from build123d import *

# Parameters (mm, degrees)
SKETCH2_R           = 90
SKETCH1_R           = 90
SHELL1_T            = -2
CUT_EXTRUDE1_START  = -50
SKETCH4_R           = 90
CUT_EXTRUDE1_DEPTH  = 50
FILLET1_R           = 10
SKETCH5_R           = 88
BOSS_EXTRUDE1_DEPTH = 2


with BuildPart() as part:
    # Sketch2 → Loft1 section 0
    with BuildSketch(Plane(origin=(0, 100, 0), x_dir=(1, 0, 0), z_dir=(0, 1, 0))):
        Circle(SKETCH2_R)
    # Sketch1 → Loft1 section 1
    with BuildSketch(Plane(origin=(0, 0, 0), x_dir=(1, 0, 0), z_dir=(0, 1, 0))):
        Circle(SKETCH1_R)
    loft()

    # Shell1
    shell1_openings = [part.faces().sort_by_distance(p)[0] for p in [
        (0, 100, 0),
    ]]
    offset(amount=SHELL1_T, openings=shell1_openings, kind=Kind.INTERSECTION)

    # Sketch4 → Cut-Extrude1 (cut)
    with BuildSketch(Plane(origin=(0, 100, 0), x_dir=(1, 0, 0), z_dir=(0, 1, 0)).offset(CUT_EXTRUDE1_START)):
        with Locations(Location((0, 0, 0), (0, 0, 270))):
            Circle(SKETCH4_R)
    extrude(amount=CUT_EXTRUDE1_DEPTH, mode=Mode.SUBTRACT)

    # Fillet1
    # the kernel refuses this fillet: 10 mm, written as the material it takes off along each edge
    with BuildSketch(Plane(origin=(0, 50, 0), x_dir=(1, 0, 0), z_dir=(0, 0, -1))) as fillet1_piece_1:
        with BuildLine():
            CenterArc((80, 6), FILLET1_R, 323.130102354, 36.869897646)
            Line((88, 0), (88.16, -0.12))
            ThreePointArc((88.16, -0.12), (89, -0.2), (90, -0.2))
            Line((90, -0.2), (90.2, 0))
            Line((90.2, 0), (90.2, 6))
            Line((90.2, 6), (90, 6))
        make_face()
    revolve(axis=Axis((0, 50, 0), (0, -1, 0)), mode=Mode.SUBTRACT)

    # Sketch5 → Boss-Extrude1 (add)
    with BuildSketch(Plane(origin=(0, 2, 0), x_dir=(1, 0, 0), z_dir=(0, 1, 0))):
        with Locations(Location((0, 0, 0), (0, 0, 270))):
            Circle(SKETCH5_R)
    extrude(amount=BOSS_EXTRUDE1_DEPTH)


solid = part.part
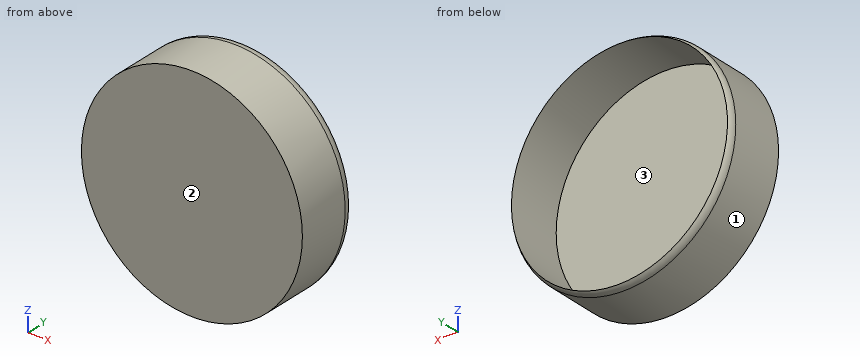
Can you work these out from the model? Positions are in its coordinate system, mm. Face numbers are marked on the shaded views. Coordinates: 2 decimals unless noted, no trailing zeros. Loops run counter-clockwise (first coordinate to the right, second up) from the corner with the lowest first, then second, coordinate; pieces in that order, holes last. Notation, with made-up numbers: M 17.5,21 L 55.5,21 A34 ccw 55.5,51 Z; hole C 11.5,23 d6. An arc over 180 degrees is marked long. Return JSON: item names as keys, results as strings. Group by question number.
Item 1: Thinking about a two-plate mould opening in X: for the marked faces 1, 2 and 3, which applies, released by +X, released by -X, zero draft, split by the parting line, or undercut?
Item 2: I'm going to push flat-ended pins straight in: pin 1 Ø3 at (y, z) = (11.5, -21.5) entering from -X; pin 2 Ø1 at (x, y) = (21, 24) entering from -Z; pin 3 Ø4 at (y, z) = (42, -20.5) entering from -X. Where does each tip first touch, or does it pass through?
Item 3: Imagine slicing it at B-B (x = 0). Please give me the cut outline in (y, z), and give its area (3 significant figures).
Item 4: If I drill on L1, parallel to Z at x = 0, y = 15.5; L2, parallel to Y at x = -45.5, z = -71; L3, parallel to X at y = 33, z = -12, over which ranges is the centre line in solid material (lowest first)? Write a range as from..to.
Item 5: Imagine slicing it at A-A (y = 38). Please give me the cut outline in (x, z).
Verdict:
{
 "1": {"face 1": "split by the parting line", "face 2": "zero draft", "face 3": "undercut"},
 "2": {"pin 1": "stops at x = -87.75", "pin 2": "stops at z = -87.63", "pin 3": "stops at x = -88.08"},
 "3": {"outline": "M 0,-90 L 44,-90 A10 ccw 50,-88 L 4,-88 L 4,88 L 50,88 A10 ccw 44,90 L 0,90 Z", "area": "896 mm^2"},
 "4": {"L1": "z = -90..-88, 88..90", "L2": "y = 0..4", "L3": "x = -89.2..-87.18, 87.18..89.2"},
 "5": {"outline": "C 0,0 d180; hole C 0,0 d176"}
}
